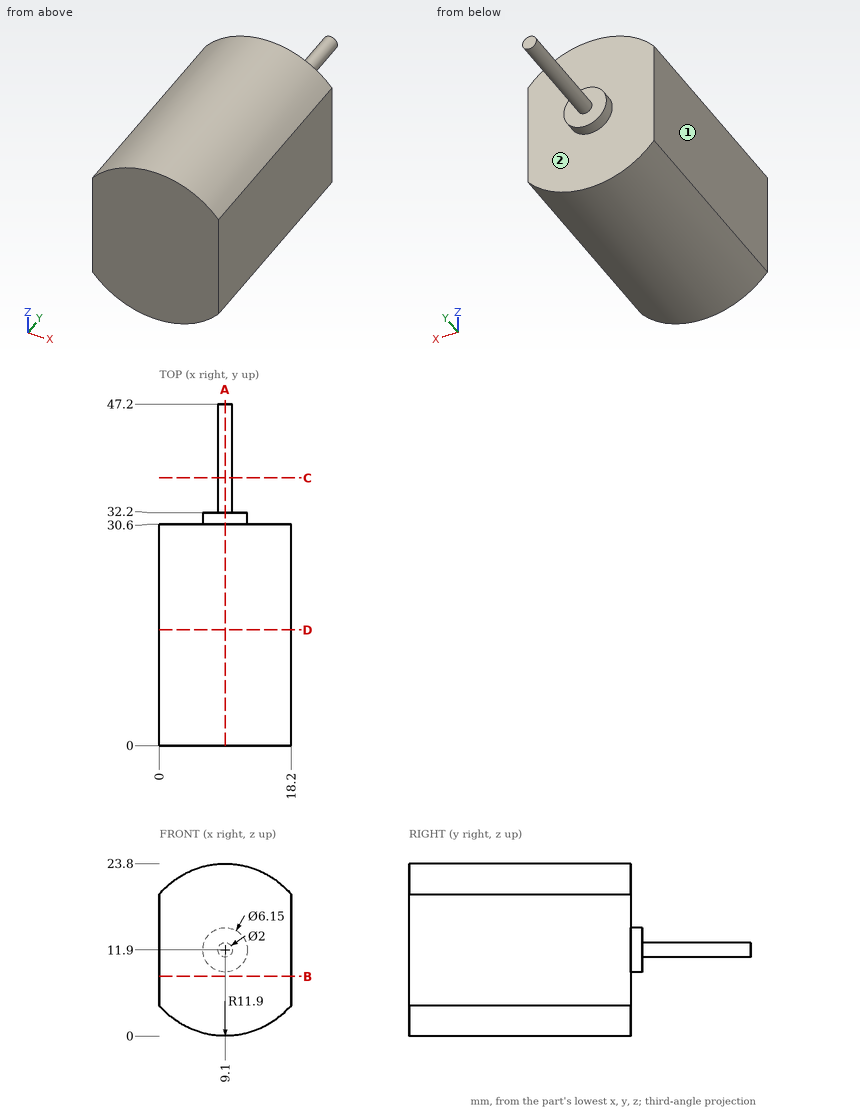
Job drawing, mm, ordinate dimensions from the low corner. One solid piece. A direction names the side the tool comes from. Coordinates: 2 decimals unless noted, no trailing zeros. Order: outer loops, then holes, each group sorted by start corner. A loop starts at its lowest first (then second) coordinate and runs counter-clockwise, first axis right, second up. Notation, with made-up numbers: (65, 13) -> (95, 13) arc R13 cw to (95, 37) -> close; hole circle Ø4 at (-15, 44.5). An arc over 180 degrees is marked (long way). Put each result on its own line as item: value. Start each with the question number.
(1) Probe line 1 along Y through (x, z) = (2, 8.75); line 2 along Y through (x, z) = (7, 11); line 3 along X through (y, z) = (37, 12) (3 decimals). List the from-to ranges inside material, lowest first. Write a range as [from, to].
(2) Which spindle directions (+Z, -Z, +X, -X, +Y, -Y) get a long thin tool onto all of the face, cutting with end or side? Do the marked faces 1 and 2. Say none if no direction does.
(3) Pin check, flat tips, straight feed: pin 1 Ø1 at (x, y) = (8, 22) entering from -Z; pin 2 Ø3 at (x, y) = (15, 24.5) entering from +Z. Stop position of each tip, or through.
(4) Band-saw the part on C-C (y = 37). Give the cut face in (x, z), then the cut area to 3 significant figures.
(5) Band-saw the part on B-B (z = 8.25). Give the cut face in (x, y), then the cut area to 3 significant figures.
(6) Band-saw the part on D-D (y = 16). Give the cut face in (x, z), then the cut area to 3 significant figures.
(7) Band-saw the part on A-A (x = 9.1). Give the cut face in (y, z) (3 decimals).
Determined:
1. line 1: y = [0, 30.6]
1. line 2: y = [0, 32.2]
1. line 3: x = [8.105, 10.095]
2. face 1: +Z, -Z, -X, +Y, -Y
2. face 2: +Y
3. pin 1: stops at z = 0.02
3. pin 2: stops at z = 22.96
4. outline: circle Ø2 at (9.1, 11.9)
4. area: 3.14 mm²
5. outline: (0, 0) -> (18.2, 0) -> (18.2, 30.6) -> (0, 30.6) -> close
5. area: 557 mm²
6. outline: (0, 4.23) arc R11.9 ccw to (18.2, 4.23) -> (18.2, 19.57) arc R11.9 ccw to (0, 19.57) -> close
6. area: 386 mm²
7. outline: (0, 0) -> (30.6, 0) -> (30.6, 8.825) -> (32.2, 8.825) -> (32.2, 10.9) -> (47.2, 10.9) -> (47.2, 12.9) -> (32.2, 12.9) -> (32.2, 14.975) -> (30.6, 14.975) -> (30.6, 23.8) -> (0, 23.8) -> close
